from build123d import *

# Parameters (mm, degrees)
F1_DEPTH = 2.54
F3_DEPTH = 6.35
F4_W     = 78.105
F4_H     = 205.105
F5_DEPTH = 3.81
F6_W     = 73.025
F6_H     = 200.025
F7_DEPTH = 2.54


with BuildPart() as f1:
    # F0 (on Top) → F1 (new body)
    with BuildSketch(Plane.XY):
        with BuildLine():
            ThreePointArc((0, 1.27), (0.371974, 0.371974), (1.27, 0))
            Line((1.27, 0), (89.535, 0))
            ThreePointArc((89.535, 0), (90.433026, 0.371974), (90.805, 1.27))
            Line((90.805, 1.27), (90.805, 216.535))
            ThreePointArc((90.805, 216.535), (90.433026, 217.433026), (89.535, 217.805))
            Line((89.535, 217.805), (1.27, 217.805))
            ThreePointArc((1.27, 217.805), (0.371974, 217.433026), (0, 216.535))
            Line((0, 216.535), (0, 1.27))
        make_face()
    extrude(amount=F1_DEPTH)

    # F2 (on Top) → F3 (join)
    with BuildSketch(Plane.XY):
        with BuildLine():
            Line((3.81, 212.725), (3.81, 5.08))
            ThreePointArc((3.81, 5.08), (4.181974, 4.181974), (5.08, 3.81))
            Line((5.08, 3.81), (85.725, 3.81))
            ThreePointArc((85.725, 3.81), (86.623026, 4.181974), (86.995, 5.08))
            Line((86.995, 5.08), (86.995, 212.725))
            ThreePointArc((86.995, 212.725), (86.623026, 213.623026), (85.725, 213.995))
            Line((85.725, 213.995), (5.08, 213.995))
            ThreePointArc((5.08, 213.995), (4.181974, 213.623026), (3.81, 212.725))
        make_face()
    extrude(amount=F3_DEPTH)

    # F4 (on face) → F5 (cut)
    with BuildSketch(Plane.XY.offset(6.35)):
        with Locations((45.4025, 108.9025)):
            Rectangle(F4_W, F4_H)
    extrude(amount=-F5_DEPTH, mode=Mode.SUBTRACT)

    # F6 (on face) → F7 (cut)
    with BuildSketch(Plane.XY.offset(2.54)):
        with Locations((45.4025, 108.9025)):
            Rectangle(F6_W, F6_H)
    extrude(amount=-F7_DEPTH, mode=Mode.SUBTRACT)


solid = f1.part
Here's how the part is built. I have some questions about the finished solid (model axes, mm). A direction names the side the tool comes from. Coordinates: 2 decimals unless noted, no trailing zeros. Order: outer loops, then holes, each group sorted by start corner. A loop starts at its lowest first (then second) coordinate and runs counter-clockwise, first axis right, second up. Notation, with made-up numbers: M 44,0.5 L 98,0.5 A33 ccw 98,36.5 Z; hole C 65,-39.5 d6. An arc over 180 degrees is marked long. Answer as CSV lines item,"result". Start each with the question number.
1. On a 3-axis mill with a long thin cutter (end or side, diameter ignored), from which of +Z, -Z, +X, -X, +Y, -Y can I reach the whole of each face in a straight line? I mean faces 4 (the flat face through (8, 117, 0)), 5 (the flat face through (86.995, 107, 4)), 6 (the flat face through (6.35, 107, 4)), 7 (the flat face through (45, 3.81, 4)). Say none if no direction works.
2. We'd pull the mould along X, two halves only. Please class faces 1 (the flat face through (84.455, 107, 4)), 2 (the flat face through (3.81, 110, 4)), 3 (the flat face through (46, 213.995, 4)): released by +X, released by -X, zero draft, split by the parting line, or undercut.
3. I want a section at C-C, the plane z = 3.5. Write out the boundary of the cut face in (x, y) (3 decimals).
4. For pin 1 (1.1 mm diameter, centred on x = 44, z = 5, fed in from -Y); pin 2 (1.1 mm diameter, centred on y = 102.5, z = 5, fed in from +X) (3 decimals); pin 3 (1.1 mm diameter, centred on y = 100.5, z = 4.5, fed in from -X), each with a flat end and sliding along its axis, tell me the tip position at first contact or that it passes through.
5. I want a section at B-B, the plane x = 78. Write out the boundary of the cut face in (y, z) (3 decimals).
6. I need wall thicknesses on line 1 (X direction, y = 61, z = 4.25) (3 decimals); line 2 (Y direction, x = 33.5, z = 0.5) (3 decimals); line 3 (X direction, y = 206, z = 1.5) (3 decimals). Which ranges of each line are inside material? Lowest first, please. Write a range as [from, to].
7. I want a section at A-A, the plane y = 193. Write out the boundary of the cut face in (x, z) (3 decimals), and give its area (3 significant figures).
Recorded:
1,face 4,"-Z, +X, -X, +Y, -Y"
1,face 5,"+Z, +X, +Y, -Y"
1,face 6,"+Z"
1,face 7,"+Z, +X, -X, -Y"
2,face 1,"undercut"
2,face 2,"released by -X"
2,face 3,"zero draft"
3,outline,"M 3.81,5.08 A1.27 ccw 5.08,3.81 L 85.725,3.81 A1.27 ccw 86.995,5.08 L 86.995,212.725 A1.27 ccw 85.725,213.995 L 5.08,213.995 A1.27 ccw 3.81,212.725 Z; hole M 6.35,6.35 L 84.455,6.35 L 84.455,211.455 L 6.35,211.455 Z"
4,pin 1,"stops at y = 3.81"
4,pin 2,"stops at x = 86.995"
4,pin 3,"stops at x = 3.81"
5,outline,"M 0,0 L 8.89,0 L 8.89,2.54 L 6.35,2.54 L 6.35,6.35 L 3.81,6.35 L 3.81,2.54 L 0,2.54 Z; M 208.915,0 L 217.805,0 L 217.805,2.54 L 213.995,2.54 L 213.995,6.35 L 211.455,6.35 L 211.455,2.54 L 208.915,2.54 Z"
6,line 1,"x = [3.81, 6.35], [84.455, 86.995]"
6,line 2,"y = [0, 8.89], [208.915, 217.805]"
6,line 3,"x = [0, 8.89], [81.915, 90.805]"
7,outline,"M 0,0 L 8.89,0 L 8.89,2.54 L 6.35,2.54 L 6.35,6.35 L 3.81,6.35 L 3.81,2.54 L 0,2.54 Z; M 81.915,0 L 90.805,0 L 90.805,2.54 L 86.995,2.54 L 86.995,6.35 L 84.455,6.35 L 84.455,2.54 L 81.915,2.54 Z"
7,area,"64.5 mm2"
